Can you work these out from the model? Positions are in its coordinate system, mm. Face numbers are marked on the shaded views. A direction names the side the tool comes from. Give positions to 0.01 mm unless a question says otherwise; leave off trailing zeros. Answer as CSV lines item,"result".
```python
from build123d import *

# Parameters (mm, degrees)
SKETCH2_R           = 2.1
CUT_EXTRUDE1_DEPTH  = 2
SKETCH4_R           = 1.95
BOSS_EXTRUDE2_DEPTH = 2.5
BOSS_EXTRUDE2_TAPER = 1


with BuildPart() as part:
    # Sketch1 → Revolve1 (revolve)
    with BuildSketch(Plane.XY, mode=Mode.PRIVATE) as revolve1_sk:
        with BuildLine():
            Line((0, -2), (-2, -2))
            Line((-2, -2), (-2, 0))
            Line((-2, 0), (-3.75, 0))
            Line((-3.75, 0), (-3.75, 0.506327417))
            add(Edge.make_bspline(
                [(-0.247423506, 6.752576494), (-1.479776467, 4.708862861), (-3.282918319, 2.94887927), (-3.75, 0.506327417)],
                knots=[0, 0, 0, 0, 1, 1, 1, 1], degree=3))
            Line((-0.247423506, 6.752576494), (0, 7))
            Line((0, 7), (0, -2))
        make_face()
    revolve(revolve1_sk.sketch.rotate(Axis((0, -2, 0), (0, 1, 0)), 270), axis=Axis((0, -2, 0), (0, 1, 0)))

    # Sketch2 → Cut-Extrude1 (cut)
    with BuildSketch(Plane.XZ.offset(2)):
        Circle(SKETCH2_R)
    extrude(amount=-CUT_EXTRUDE1_DEPTH, mode=Mode.SUBTRACT)

    # Sketch4 → Boss-Extrude2 (add)
    with BuildSketch(Plane.XZ):
        Circle(SKETCH4_R)
    extrude(amount=BOSS_EXTRUDE2_DEPTH, taper=BOSS_EXTRUDE2_TAPER)


solid = part.part
```
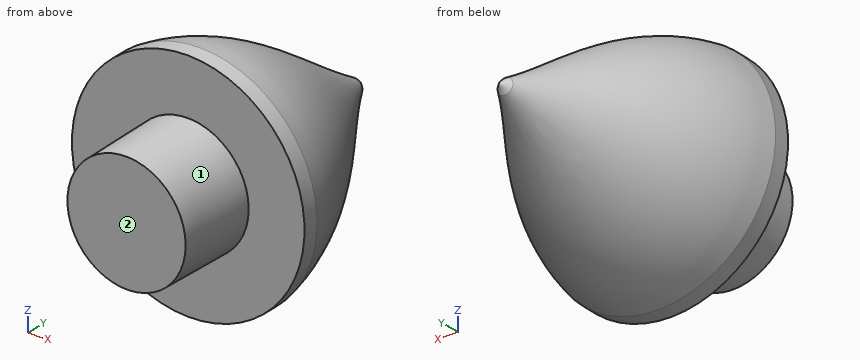
1) I need wall thicknesses on line 1 along Z through (x, y) = (-0.25, 0.5); line 2 along Y through (x, z) = (2.25, -0.75); line 3 along Y through (x, z) = (0.25, -0.5). Which ranges of each line are inside material? Lowest first, please. Write a range as [from, to].
Answer block:
line 1,"[-3.74, 3.74]"
line 2,"[0, 3.65]"
line 3,"[-2.5, 6.26]"
2) I'm going to push flat-ended pins straight in: P1, Ø3, axis at x = -2.5, z = 1.5, coming from the +Y side; P2, Ø1, axis at x = -1, y = 4, coming from the +Z side; P3, Ø1.5, axis at y = 3, z = 2.5, coming from the -X side. Where does each tip first touch, or does it pass through?
Answer block:
P1,"y = 5.02"
P2,"z = 2.31"
P3,"x = -2.35"
3) Which directions (+Z, -Z, +X, -X, +Y, -Y) give clear straight access to the entire face, cutting with the end or side of a thin tool? Please do the marked faces 1 and 2.
Answer block:
face 1,"-Y"
face 2,"+Z, -Z, +X, -X, -Y"
